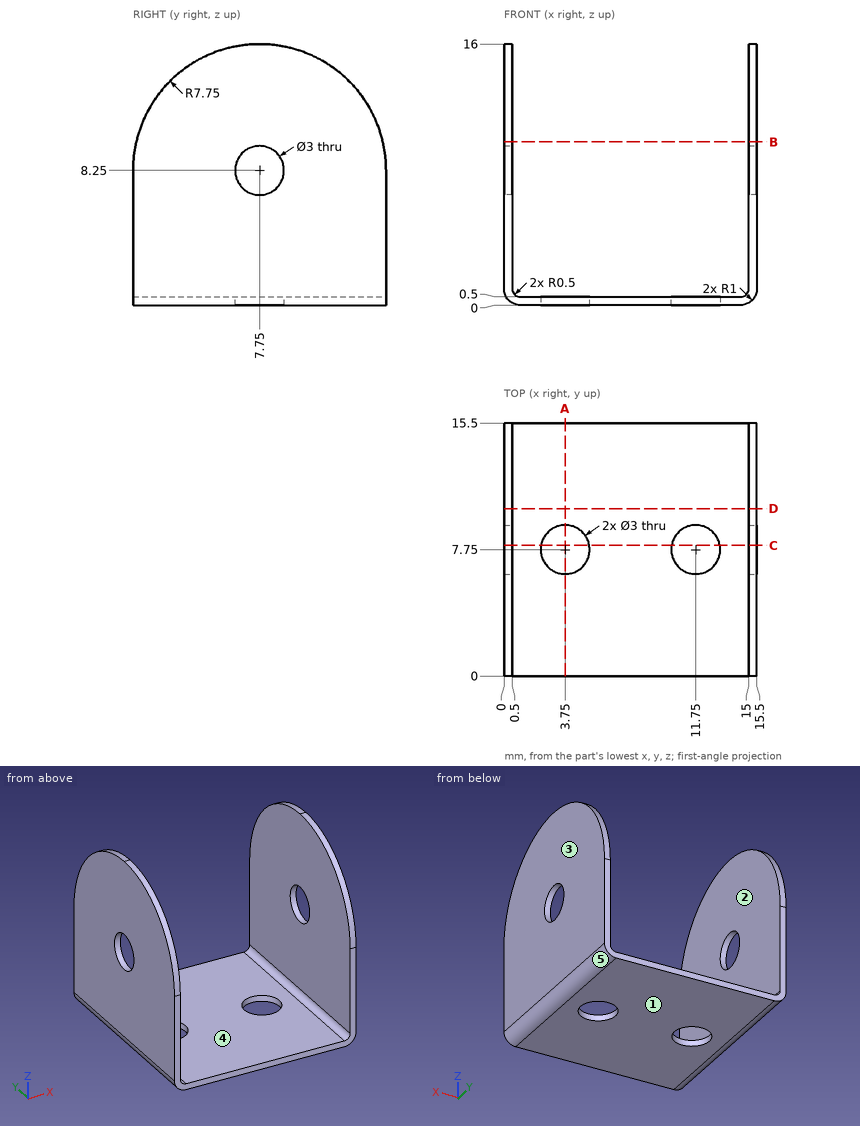
Source: three-view drawing plus pictorial views. Frame: mm from the lowest corner of the part. A direction names the side the tool comes from. Round coordinates to 2 decimals unless told otherwise and drop trailing zeros. Order: outer loops, then holes, each group sorted by start corner. A loop starts at its lowest first (then second) coordinate and runs counter-clockwise, first axis right, second up. Notation, with made-up numbers: (12.25, 86.5) - (33.25, 86.5) arc R22 ccw to (33.25, 122.5) - close; hole circle Ø2 at (13.25, 44). An arc over 180 degrees is marked (long way). Use a Markdown table: item, result.
1. Mould query, pull axis X, two halves, no side actions, for the marked faces 1, 2 and 3. Classes: +X half, -X half, draft (parallel to the pull), parting line (faces both ways), or undercut.
Evaluation:
| item | result |
|---|---|
| face 1 | draft |
| face 2 | undercut |
| face 3 | +X half |
2. Section B-B on z = 10. Return the cut outline in (x, y).
Evaluation:
| item | result |
|---|---|
| outline | (0, 0.2) - (0.5, 0.2) - (0.5, 15.3) - (0, 15.3) - close; (15, 0.2) - (15.5, 0.2) - (15.5, 15.3) - (15, 15.3) - close |
3. Section D-D on y = 10.25. Return the cut outline in (x, z), then the cut area to 3 significant figures.
Evaluation:
| item | result |
|---|---|
| outline | (0, 1) arc R1 ccw to (1, 0) - (14.5, 0) arc R1 ccw to (15.5, 1) - (15.5, 15.59) - (15, 15.59) - (15, 1) arc R0.5 cw to (14.5, 0.5) - (1, 0.5) arc R0.5 cw to (0.5, 1) - (0.5, 15.59) - (0, 15.59) - close |
| area | 22.5 mm^2 |
4. Section C-C on y = 8. Return the cut outline in (x, z).
Evaluation:
| item | result |
|---|---|
| outline | (0, 1) arc R1 ccw to (1, 0) - (2.27, 0) - (2.27, 0.5) - (1, 0.5) arc R0.5 cw to (0.5, 1) - (0.5, 6.77) - (0, 6.77) - close; (0, 9.73) - (0.5, 9.73) - (0.5, 16) - (0, 16) - close; (5.23, 0) - (10.27, 0) - (10.27, 0.5) - (5.23, 0.5) - close; (13.23, 0) - (14.5, 0) arc R1 ccw to (15.5, 1) - (15.5, 6.77) - (15, 6.77) - (15, 1) arc R0.5 cw to (14.5, 0.5) - (13.23, 0.5) - close; (15, 9.73) - (15.5, 9.73) - (15.5, 16) - (15, 16) - close |
5. Material intervals for probe 1 along Y at (x, z) = (3.75, 0.2); probe 2 along X at (y, z) = (4, 14.75); probe 3 along Z at (x, y) = (8.25, 2.5), sorted ascending.
Evaluation:
| item | result |
|---|---|
| probe 1 | 0 to 6.25, 9.25 to 15.5 |
| probe 2 | 0 to 0.5, 15 to 15.5 |
| probe 3 | 0 to 0.5 |
6. Access query for the marked faces 4 and 5. Directions: +Z, -Z, +X, -X, +Y, -Y. A direction counts if a zero-diameter tool reaches every point of the face in a straight line with its end or side. Return the directions, or none.
Evaluation:
| item | result |
|---|---|
| face 4 | +Z, +Y, -Y |
| face 5 | -Z, +X, +Y, -Y |
7. First-contact query: pin 1 (5 mm diameter, centred on x = 3.75, y = 7.75, fed in from +Z). Flat tip, straight axial feed; report the tip coordinate or a pass-through.
Evaluation:
| item | result |
|---|---|
| pin 1 | z = 0.5 |
8. Section A-A on x = 3.75. Return the cut outline in (y, z), then the cut area to 3 significant figures.
Evaluation:
| item | result |
|---|---|
| outline | (0, 0) - (6.25, 0) - (6.25, 0.5) - (0, 0.5) - close; (9.25, 0) - (15.5, 0) - (15.5, 0.5) - (9.25, 0.5) - close |
| area | 6.25 mm^2 |
